```python
from build123d import *

# Parameters (mm, degrees)
F0_W     = 8
F0_H     = 3.7
F1_DEPTH = 56
F3_W     = 56
F3_H     = 39
F4_DEPTH = 1.8
F5_DEPTH = 25
F6_R     = 1
F7_R     = 1.5
F8_R     = 1
F9_DEPTH = 2


with BuildPart() as f1:
    # F0 (on Right) → F1 (new body)
    with BuildSketch(Plane.YZ):
        Polygon((-1.5, 0), (0, 0), (0, 9), (-19.5, 9), (-19.5, 5.3), (-19.5, 0), (-12.5, 0), (-12, 6), (-2, 6), align=None)
        with Locations((-23.5, 7.15)):
            Rectangle(F0_W, F0_H)
        Polygon((0, 9), (0, 0), (1.5, 0), (2, 6), (12, 6), (12.5, 0), (19.5, 0), (19.5, 5.3), (19.5, 9), align=None)
        with Locations((23.5, 7.15)):
            Rectangle(F0_W, F0_H)
    extrude(amount=F1_DEPTH)

    # F3 (on face) → F4 (join)
    with BuildSketch(Plane.XY.offset(9)):
        with Locations((28, 0)):
            Rectangle(F3_W, F3_H)
    extrude(amount=F4_DEPTH)

    # F2 (on face) → F5 (cut)
    with BuildSketch(Plane.XY.offset(9)):
        with BuildLine():
            Line((11.5, -27.5), (11.5, -23.5))
            ThreePointArc((11.5, -23.5), (10, -25), (8.5, -23.5))
            Line((8.5, -23.5), (8.5, -27.5))
            Line((8.5, -27.5), (11.5, -27.5))
        make_face()
        with BuildLine():
            ThreePointArc((8.5, -23.5), (10, -25), (11.5, -23.5))
            ThreePointArc((11.5, -23.5), (10, -22), (8.5, -23.5))
        make_face()
        with BuildLine():
            Line((44.5, -23.5), (44.5, -27.5))
            Line((44.5, -27.5), (47.5, -27.5))
            Line((47.5, -27.5), (47.5, -23.5))
            ThreePointArc((47.5, -23.5), (46, -25), (44.5, -23.5))
        make_face()
        with BuildLine():
            ThreePointArc((47.5, -23.5), (46, -22), (44.5, -23.5))
            ThreePointArc((44.5, -23.5), (46, -25), (47.5, -23.5))
        make_face()
        with BuildLine():
            Line((11.5, 27.5), (8.5, 27.5))
            Line((8.5, 27.5), (8.5, 23.5))
            ThreePointArc((8.5, 23.5), (10, 25), (11.5, 23.5))
            Line((11.5, 23.5), (11.5, 27.5))
        make_face()
        with BuildLine():
            ThreePointArc((11.5, 23.5), (10, 25), (8.5, 23.5))
            ThreePointArc((8.5, 23.5), (10, 22), (11.5, 23.5))
        make_face()
        with BuildLine():
            ThreePointArc((44.5, 23.5), (46, 22), (47.5, 23.5))
            ThreePointArc((47.5, 23.5), (46, 25), (44.5, 23.5))
        make_face()
        with BuildLine():
            Line((47.5, 23.5), (47.5, 27.5))
            Line((47.5, 27.5), (44.5, 27.5))
            Line((44.5, 27.5), (44.5, 23.5))
            ThreePointArc((44.5, 23.5), (46, 25), (47.5, 23.5))
        make_face()
    extrude(amount=-F5_DEPTH, mode=Mode.SUBTRACT)

    # F6
    f6_edges = [f1.edges().sort_by_distance(p)[0] for p in [
        (56, 19.5, 2.65),
        (56, 12.25, 3),
        (56, 1.75, 3),
        (56, -1.75, 3),
        (56, -12.25, 3),
        (56, -19.5, 2.65),
        (56, 19.5, 9.9),
        (56, -19.5, 9.9),
        (0, 19.5, 2.65),
        (0, 12.25, 3),
        (0, 1.75, 3),
        (0, -1.75, 3),
        (0, 19.5, 9.9),
        (0, -12.25, 3),
        (0, -19.5, 2.65),
        (0, -19.5, 9.9),
    ]]
    fillet(f6_edges, radius=F6_R)

    # F7
    f7_edges = [f1.edges().sort_by_distance(p)[0] for p in [
        (0, -27.5, 7.15),
        (8.5, -27.5, 7.15),
        (11.5, -27.5, 7.15),
        (47.5, -27.5, 7.15),
        (44.5, -27.5, 7.15),
        (56, -27.5, 7.15),
        (0, 27.5, 7.15),
        (8.5, 27.5, 7.15),
        (11.5, 27.5, 7.15),
        (44.5, 27.5, 7.15),
        (47.5, 27.5, 7.15),
        (56, 27.5, 7.15),
    ]]
    fillet(f7_edges, radius=F7_R)

    # F8 (on face) → F9 (join)
    with BuildSketch(Plane(origin=(0, 0, 0), x_dir=(1, 0, 0), z_dir=(0, 0, -1))):
        with Locations((38, 0)):
            Circle(F8_R)
        with Locations((18, 0)):
            Circle(F8_R)
        with Locations((26.9247623258, 16.2018900485)):
            Circle(F8_R)
        with Locations((27.9158912599, -15.5527964234)):
            Circle(F8_R)
    extrude(amount=F9_DEPTH)


solid = f1.part
```
Design review of the part built by this model. Coordinates are the model's own, in mm. A direction names the side the tool comes from. Coordinates: 2 decimals unless noted, no trailing zeros. Loops run counter-clockwise (first coordinate to the right, second up) from the corner with the lowest first, then second, coordinate; pieces in that order, holes last.
Q1. We need section D-D on x = 30. State the section outline as (y, z) points.
Reported:
outline: (-27.5, 5.3) - (-19.5, 5.3) - (-19.5, 0) - (-12.5, 0) - (-12, 6) - (-2, 6) - (-1.5, 0) - (1.5, 0) - (2, 6) - (12, 6) - (12.5, 0) - (19.5, 0) - (19.5, 5.3) - (27.5, 5.3) - (27.5, 9) - (19.5, 9) - (19.5, 10.8) - (-19.5, 10.8) - (-19.5, 9) - (-27.5, 9) - close
Q2. We need section C-C on z = 3.75. State how many separate pieces and enclosed holes the cut face has, and give its area (3 significant figures).
Reported:
separate pieces: 3
enclosed holes: 0
area: 1,020 mm2
Q3. Tool access review of faces 5 (the face through (0.285, 12.557, 2.941)), 6 (the face through (11.93, 27.05, 7.12)), 7 (the face through (28, 19.5, 3)): name each direction out of +Z, -Z, +X, -X, +Y, -Y from which nothing blocks a thin tool from reaching the whole face with its end or side.
Reported:
face 5: -Z, -X
face 6: +Z, -Z, +Y
face 7: -Z, +X, -X, +Y
Q4. We need section A-A on x = 46. State the section outline as (y, z) points.
Reported:
outline: (-22, 5.3) - (-19.5, 5.3) - (-19.5, 0) - (-12.5, 0) - (-12, 6) - (-2, 6) - (-1.5, 0) - (1.5, 0) - (2, 6) - (12, 6) - (12.5, 0) - (19.5, 0) - (19.5, 5.3) - (22, 5.3) - (22, 9) - (19.5, 9) - (19.5, 10.8) - (-19.5, 10.8) - (-19.5, 9) - (-22, 9) - close
Q5. The part is to be moulded in two halves that separate along Y. For faces 1 (the face through (28, -27.5, 7)), 2 (the face through (38, 0, -2)), 3 (the face through (27.622, 12.246, 3.042)), 4 (the face through (44.05, 27.07, 7.12)), say which applies: +Y half, -Y half, draft (parallel to the pull), parting line (faces both ways), or undercut.
Reported:
face 1: -Y half
face 2: draft
face 3: undercut
face 4: +Y half
Q6. For pin 1 (2.5 mm diameter, centred on x = 33, z = 3.5, fed in from -Y); pin 2 (13 mm diameter, centred on x = 29.5, y = 7.5, fed in from -Z); pin 3 (4.5 mm diameter, centred on x = 15.5, y = 25, fed in from -Z), all flat-tipped, find the tip position at first contact; note any pin that passes through.
Reported:
pin 1: stops at y = -19.5
pin 2: stops at z = 0
pin 3: stops at z = 5.3
Q7. We need section B-B on y = 8.5. State the section outline as (x, z) points, and give its area (3 significant figures).
Reported:
outline: (0, 6) - (56, 6) - (56, 10.8) - (0, 10.8) - close
area: 269 mm2
Q8. To check wall thickness, follow line 1 (X direction, y = 24.5, z = 7); line 2 (Y direction, x = 50, z = 5.25); line 3 (Y direction, x = 52, z = 3.75). State the ranges of each line that lie inside material, in increasing order.
Reported:
line 1: x = 0 to 8.5, 11.5 to 44.5, 47.5 to 56
line 2: y = -19.5 to -12.06, -1.94 to 1.94, 12.06 to 19.5
line 3: y = -19.5 to -12.19, -1.81 to 1.81, 12.19 to 19.5
